from build123d import *

# Parameters (mm, degrees)
BOSS_EXTRUDE1_DEPTH = 130
SKETCH2_R           = 48
CUT_EXTRUDE1_DEPTH  = 3
SKETCH3_R           = 1.9
CUT_EXTRUDE2_DEPTH  = 3
BOSS_EXTRUDE2_DEPTH = 3
BOSS_EXTRUDE3_DEPTH = 3
SKETCH6_R           = 2
CUT_EXTRUDE3_DEPTH  = 3


with BuildPart() as part:
    # Sketch1 → Boss-Extrude1 (new body)
    with BuildSketch(Plane(origin=(0, 0, 0), x_dir=(0, 0, -1), z_dir=(1, 0, 0))):
        Polygon((-3, 126), (169, -3), (-3, -3), align=None)
        Polygon((0, 0), (160, 0), (0, 120), align=None, mode=Mode.SUBTRACT)
    extrude(amount=BOSS_EXTRUDE1_DEPTH)

    # Sketch2 → Cut-Extrude1 (cut)
    with BuildSketch(Plane(origin=(0, 79.2, -59.4), x_dir=(1, 0, 0), z_dir=(0, 0.7999999999999998, -0.6000000000000002))):
        with Locations(Location((65, 10, 0), (0, 0, 270))):
            Circle(SKETCH2_R)
    extrude(amount=-CUT_EXTRUDE1_DEPTH, mode=Mode.SUBTRACT)

    # Sketch3 → Cut-Extrude2 (cut)
    with BuildSketch(Plane(origin=(0, 79.2, -59.4), x_dir=(1, 0, 0), z_dir=(0, 0.7999999999999998, -0.6000000000000002))):
        with Locations(Location((11, 10, 0), (0, 0, 270))):
            Circle(SKETCH3_R)
        with Locations(Location((65, -44, 0), (0, 0, 270))):
            Circle(SKETCH3_R)
        with Locations(Location((119, 10, 0), (0, 0, 270))):
            Circle(SKETCH3_R)
        with Locations(Location((65, 64, 0), (0, 0, 270))):
            Circle(SKETCH3_R)
    extrude(amount=-CUT_EXTRUDE2_DEPTH, mode=Mode.SUBTRACT)

    # Sketch4 → Boss-Extrude2 (add)
    with BuildSketch(Plane(origin=(130, 0, 0), x_dir=(0, 0, -1), z_dir=(1, 0, 0))):
        Polygon((-3, -3), (-3, 126), (169, -3), align=None)
    extrude(amount=BOSS_EXTRUDE2_DEPTH)

    # Sketch5 → Boss-Extrude3 (add)
    with BuildSketch(Plane.ZY):
        Polygon((3, 126), (3, -3), (-169, -3), align=None)
    extrude(amount=BOSS_EXTRUDE3_DEPTH)

    # Sketch6 → Cut-Extrude3 (cut)
    with BuildSketch(Plane.XY.offset(3)):
        with Locations((65, 21.56057542)):
            Circle(SKETCH6_R)
    extrude(amount=-CUT_EXTRUDE3_DEPTH, mode=Mode.SUBTRACT)


solid = part.part
Design review of the part built by this model. Coordinates are the model's own, in mm. A direction names the side the tool comes from. Coordinates: 2 decimals unless noted, no trailing zeros. Order: outer loops, then holes, each group sorted by start corner. A loop starts at its lowest first (then second) coordinate and runs counter-clockwise, first axis right, second up. Notation, with made-up numbers: (51, -17) -> (100, -17) arc R7 ccw to (100, -12) -> close; hole circle Ø8 at (-37, 59). An arc over 180 degrees is marked (long way). One line per item, written item: value.
1) Clearance check with flat-ended pins moving along their axes: P1, Ø3.5, axis at x = 65, y = 21.56, coming from the -Z side; P2, Ø1.5, axis at x = 33.5, z = -38, coming from the +Y side; P3, Ø1.5, axis at x = 49, z = -28.5, coming from the +Y side. State where each tip first meets the part, or that it passes through.
Output values:
P1: stops at z = -138.59
P2: stops at y = 95.81
P3: stops at y = 102.94
2) Draft analysis for pull direction Z (two halves, no side actions). For faces 4 (the face through (66, -3, -82)), 5 (the face through (66, 62, 3)), 6 (the face through (64, 0, -79)), state which applies: +Z half, -Z half, draft (parallel to the pull), parting line (faces both ways), or undercut.
Output values:
face 4: draft
face 5: +Z half
face 6: undercut
3) Machinability: for faces 1 (the face through (64.74, 23.544, 1.521)), 2 (the face through (-3, 34, -44)), 3 (the face through (64, 61, 0)), which of the approach directions +Z, -Z, +X, -X, +Y, -Y give a long, thin tool a straight path to every point of the face, cutting with its end or side? Answer none if there is none.
Output values:
face 1: +Z
face 2: +Z, -Z, -X, +Y, -Y
face 3: none
4) We need section B-B, the plane y = 26.5. Give the boundary of the cut face in (x, z), then the cut area to 3 significant figures.
Output values:
outline: (-3, -129.67) -> (133, -129.67) -> (133, 3) -> (-3, 3) -> close; hole (0, -124.67) -> (130, -124.67) -> (130, 0) -> (0, 0) -> close
area: 1,840 mm2
5) We need section A-A, the plane z = -122. Give the boundary of the cut face in (x, y).
Output values:
outline: (-3, -3) -> (133, -3) -> (133, 32.25) -> (-3, 32.25) -> close; hole (0, 0) -> (130, 0) -> (130, 28.5) -> (0, 28.5) -> close
6) To check wall thickness, follow probe 1 along X at (y, z) = (43.5, -52.5); probe 2 along Z at (x, y) = (39, 73.5); probe 3 along Y at (x, z) = (40, -71). State the ranges of each line that lie inside material, in increasing order. Write a range as [from, to].
Output values:
probe 1: x = [-3, 0], [130, 133]
probe 2: z = [0, 3]
probe 3: y = [-3, 0]
7) We need section C-C, the plane x = 106.5. Give the boundary of the cut face in (y, z), then the cut area to 3 significant figures.
Output values:
outline: (-3, -169) -> (58.73, -86.7) -> (56.33, -84.9) -> (0, -160) -> (0, 0) -> (120, 0) -> (85.27, -46.3) -> (87.67, -48.1) -> (126, 3) -> (-3, 3) -> close
area: 1,350 mm2
